Geometry check sheet. Reference: the model listing, model coordinates, mm. Round coordinates to 2 decimals unless told otherwise and drop trailing zeros. Order: outer loops, then holes, each group sorted by start corner. A loop starts at its lowest first (then second) coordinate and runs counter-clockwise, first axis right, second up.
(1) Sectioned sample at B-B (y = -20). Record the boundary of the cut face in (x, z), plus the area to 3 significant figures.
(2) Material ranges on line 1 along Y through (x, z) = (0, 0.4); line 2 along X through (y, z) = (5, 2.05); line 3 along Y through (x, z) = (-7, 1.55), recorded low to high.
(3) Sectioned sample at C-C (z = 0.8). Record the boundary of the cut face in (x, y), plus the area to 3 significant figures.
(4) Sectioned sample at A-A (x = 0). Record the boundary of the cut face in (y, z).
from build123d import *

# Parameters (mm, degrees)
SKETCH1_W      = 70
SKETCH1_H      = 150
EXTRUDE1_DEPTH = 3
EXTRUDE2_REACH = 5
SKETCH2_R      = 15
EXTRUDE3_REACH = 5
SKETCH4_W      = 1.5
SKETCH4_H      = 1.5
FILLET1_R      = 1


with BuildPart() as part:
    # Sketch1 → Extrude1 (new body)
    with BuildSketch(Plane.XY):
        with Locations((0, -55)):
            Rectangle(SKETCH1_W, SKETCH1_H)
    extrude(amount=EXTRUDE1_DEPTH)

    # Sketch2 → Extrude2 (cut, up to next)
    with BuildSketch(Plane.XY.offset(3), mode=Mode.PRIVATE) as extrude2_sk1:
        with Locations((0, -20)):
            Circle(SKETCH2_R)
    extrude2_tool1 = extrude(extrude2_sk1.sketch, amount=-EXTRUDE2_REACH, mode=Mode.PRIVATE) & part.part
    add(extrude2_tool1.solids().sort_by_distance((0, -20, 3))[0], mode=Mode.SUBTRACT)

    # Sketch4 → Extrude3 (cut, up to next)
    with BuildSketch(Plane.XY.offset(3), mode=Mode.PRIVATE) as extrude3_sk1:
        with Locations((-26.25, 11.25)):
            Rectangle(SKETCH4_W, SKETCH4_H)
    extrude3_tool1 = extrude(extrude3_sk1.sketch, amount=-EXTRUDE3_REACH, mode=Mode.PRIVATE) & part.part
    add(extrude3_tool1.solids().sort_by_distance((-26.25, 11.25, 3))[0], mode=Mode.SUBTRACT)
    # Sketch4 → Extrude3 (cut, up to next)
    with BuildSketch(Plane.XY.offset(3), mode=Mode.PRIVATE) as extrude3_sk2:
        with Locations((26.25, 11.25)):
            Rectangle(SKETCH4_W, SKETCH4_H)
    extrude3_tool2 = extrude(extrude3_sk2.sketch, amount=-EXTRUDE3_REACH, mode=Mode.PRIVATE) & part.part
    add(extrude3_tool2.solids().sort_by_distance((26.25, 11.25, 3))[0], mode=Mode.SUBTRACT)

    # Fillet1
    fillet1_edges = [part.edges().sort_by_distance(p)[0] for p in [
        (35, -55, 3),
        (0, 20, 3),
        (-15, -20, 3),
        (-27, 11.25, 3),
        (-26.25, 10.5, 3),
        (-25.5, 11.25, 3),
        (-26.25, 12, 3),
        (25.5, 11.25, 3),
        (26.25, 10.5, 3),
        (27, 11.25, 3),
        (26.25, 12, 3),
        (-35, -55, 3),
        (0, -130, 3),
    ]]
    fillet(fillet1_edges, radius=FILLET1_R)


solid = part.part
Answer below:
1. outline: (-35, 0) - (-15, 0) - (-15, 2) arc R1 ccw to (-16, 3) - (-34, 3) arc R1 ccw to (-35, 2) - close; (15, 0) - (35, 0) - (35, 2) arc R1 ccw to (34, 3) - (16, 3) arc R1 ccw to (15, 2) - close
1. area: 119 mm2
2. line 1: y = -130 to -35, -5 to 20
2. line 2: x = -35 to 35
2. line 3: y = -130 to -33.27, -6.73 to 20
3. outline: (-35, -130) - (35, -130) - (35, 20) - (-35, 20) - close; hole (-27, 10.5) - (-25.5, 10.5) - (-25.5, 12) - (-27, 12) - close; hole circle Ø30 at (0, -20); hole (25.5, 10.5) - (27, 10.5) - (27, 12) - (25.5, 12) - close
3. area: 9,790 mm2
4. outline: (-130, 0) - (-35, 0) - (-35, 2) arc R1 ccw to (-36, 3) - (-129, 3) arc R1 ccw to (-130, 2) - close; (-5, 0) - (20, 0) - (20, 2) arc R1 ccw to (19, 3) - (-4, 3) arc R1 ccw to (-5, 2) - close
